The model under review builds one solid part; all positions refer to its coordinate system, in mm. A direction names the side the tool comes from. Round coordinates to 2 decimals unless told otherwise and drop trailing zeros. Write each loop counter-clockwise with the first axis right and the second up, starting at its lowest first coordinate (ties: lowest second). Pieces come first, ordered by that corner, then holes. Notation, with made-up numbers: (39, 39.25) -> (89, 39.25) arc R18 cw to (89, 47.25) -> close; hole circle Ø4 at (-32.5, -13). An arc over 180 degrees is marked (long way). Return JSON: item names as keys, results as strings. Group by question number.
1. Take a section at A-A, the plane x = 0. Write out the cut boundary in (y, z), then the cut area to 3 significant figures.
2. Tool access review of faces 4 (the cylindrical face through (3.233, -1.341, 2.754)), 5 (the cylindrical face through (2.285, 3.584, 0.246)), 6 (the flat face through (-2, -4, 3)): name each direction out of +Z, -Z, +X, -X, +Y, -Y from which nothing blocks a thin tool from reaching the whole face with its end or side.
3. Take a section at C-C, the plane z = 1.25. Write out the cut boundary in (x, y), then the cut area to 3 significant figures.
4. Mouldability with a two-part tool opening along Y and no side actions: class faces 1 (the cylindrical face through (-3, 0, 1)), 2 (the flat face through (-2, -4, 0)), 3 (the cylindrical face through (-1.08, -4.88, 1.48)) as pulls with the +Y half, pulls with the -Y half, needs draft (parallel to the pull), parting line crosses it, or undercut.
5. For line 1 along Y through (x, z) = (0, 2.75); line 2 along Y through (x, z) = (0, 0.7); line 3 along Y through (x, z) = (4, 2.4), list the stretches that pass through material, from the lowest coordinate up. Write a range as from..to.
6. Clearance check with flat-ended pins moving along their axes: P1, Ø1, axis at y = 3.5, z = 1, coming from the +X side; P2, Ø1, axis at y = 1, z = 2, coming from the -X side; P3, Ø5.5, axis at x = 0, y = 0, coming from the -Z side. State where each tip first meets the part, or that it passes through.
from build123d import *

# Parameters (mm, degrees)
SKETCH_1_R          = 5
SKETCH_1_R_2        = 3
EXTRUDE_1_DEPTH     = 3
SKETCH_2_R          = 4.25
SKETCH_2_R_2        = 3.5
CUT_EXTRUDE_1_DEPTH = 0.5


with BuildPart() as part:
    # 草图1 → 凸台-拉伸1 (new body)
    with BuildSketch(Plane.XY):
        Circle(SKETCH_1_R)
        Circle(SKETCH_1_R_2, mode=Mode.SUBTRACT)
    extrude(amount=EXTRUDE_1_DEPTH)

    # 草图2 → 切除-拉伸1 (cut)
    with BuildSketch(Plane.XY.offset(3)):
        Circle(SKETCH_2_R)
        Circle(SKETCH_2_R_2, mode=Mode.SUBTRACT)
    cut_extrude_1 = extrude(amount=-CUT_EXTRUDE_1_DEPTH, mode=Mode.SUBTRACT)

    # 镜向1: 切除-拉伸1 across plane
    add(cut_extrude_1.mirror(Plane.XY.offset(1.5)), mode=Mode.SUBTRACT)


solid = part.part
Output:
{
 "1": {"outline": "(-5, 0) -> (-4.25, 0) -> (-4.25, 0.5) -> (-3.5, 0.5) -> (-3.5, 0) -> (-3, 0) -> (-3, 3) -> (-3.5, 3) -> (-3.5, 2.5) -> (-4.25, 2.5) -> (-4.25, 3) -> (-5, 3) -> close; (3, 0) -> (3.5, 0) -> (3.5, 0.5) -> (4.25, 0.5) -> (4.25, 0) -> (5, 0) -> (5, 3) -> (4.25, 3) -> (4.25, 2.5) -> (3.5, 2.5) -> (3.5, 3) -> (3, 3) -> close", "area": "10.5 mm^2"},
 "2": {"face 4": "+Z", "face 5": "-Z", "face 6": "+Z, +X, -X, +Y, -Y"},
 "3": {"outline": "circle Ø10 at (0, 0); hole circle Ø6 at (0, 0)", "area": "50.3 mm^2"},
 "4": {"face 1": "undercut", "face 2": "needs draft", "face 3": "parting line crosses it"},
 "5": {"line 1": "y = -5..-4.25, -3.5..-3, 3..3.5, 4.25..5", "line 2": "y = -5..-3, 3..5", "line 3": "y = -3..3"},
 "6": {"P1": "stops at x = 4", "P2": "stops at x = -4.97", "P3": "passes through"}
}
